Drawing for the job (mm, zero at the part's lowest x, y, z). A direction names the side the tool comes from. Give positions to 0.01 mm unless a question says otherwise; leave off trailing zeros. Loops run counter-clockwise (first coordinate to the right, second up) from the corner with the lowest first, then second, coordinate; pieces in that order, holes last. Notation, with made-up numbers: (20, 79.25) - (76, 79.25) arc R23 cw to (76, 117.25) - close; hole circle Ø2 at (34, 83.5). An arc over 180 degrees is marked (long way). Return JSON: item names as keys, results as strings. Group by question number.
1) Drop flat-ended pins along their axis: pin 1 (4 mm diameter, centred on x = 6, z = 9.5, fed in from -Y); pin 2 (3 mm diameter, centred on x = 3, y = 3.5, fed in from -Z); pin 3 (2 mm diameter, centred on x = 1, z = 9, fed in from -Y); pin 4 (2 mm diameter, centred on x = 2.5, z = 4.5, fed in from +Y). Give the stop position or say it passes through.
2) Drill centre lines: probe 1 along X at (y, z) = (4.5, 1.5); probe 2 along Z at (x, y) = (5.25, 5.75). Where is each one in solid material? Low to high. Write a range as from..to.
3) 3-axis set-ups, long thin cutter, end or side, ignore diameter. For the marked faces 1 and 2: which of +Z, -Z, +X, -X, +Y, -Y reach the whole face in a straight line?
4) Slice it at B-B (z = 9.5). List the corners of the cut face in (x, y), and give its area (3 significant figures).
5) Slice it at A-A (x = 3.5). List the corners of the cut face in (y, z), and give its area (3 significant figures).
6) Slice it at C-C (y = 2.75). List the corners of the cut face in (x, z), and give its area (3 significant figures).
7) Slice it at D-D (x = 6). List the corners of the cut face in (y, z).
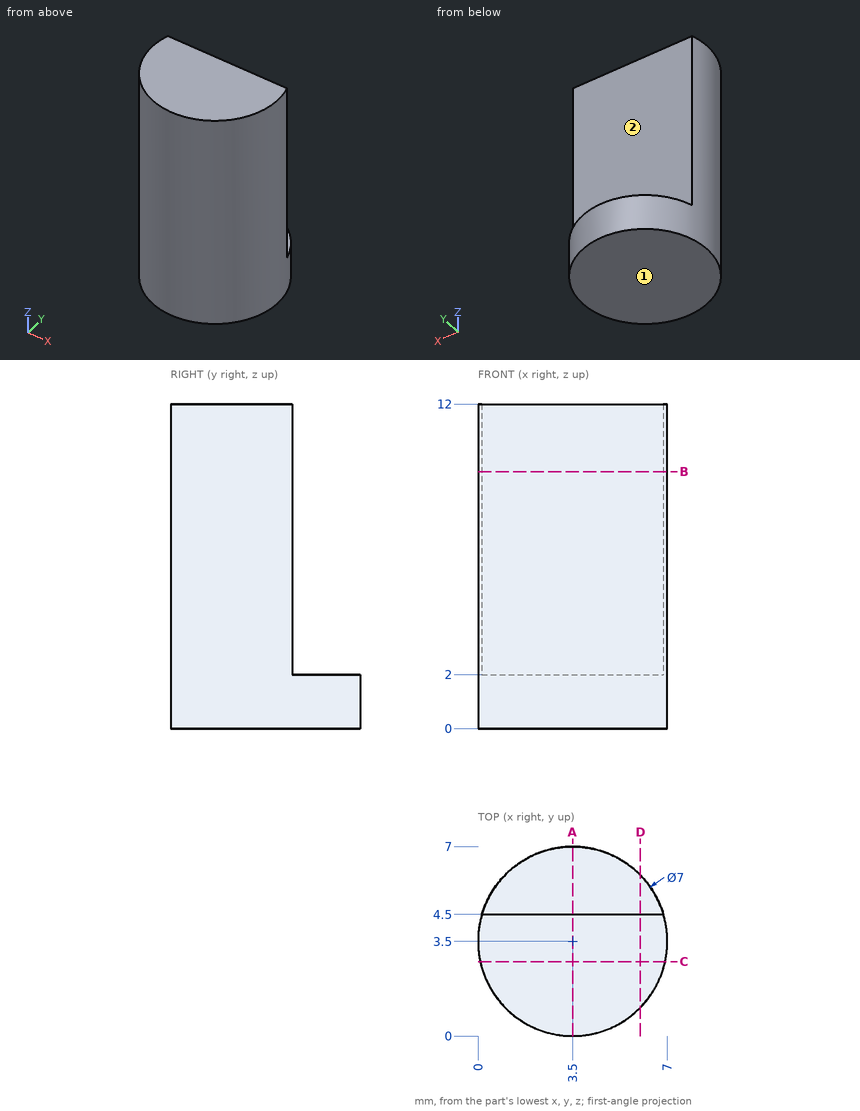
Results:
{
 "1": {"pin 1": "y = 0.04", "pin 2": "z = 0", "pin 3": "y = 0.34", "pin 4": "y = 4.5"},
 "2": {"probe 1": "0.15..6.85", "probe 2": "0..2"},
 "3": {"face 1": "-Z, +X, -X, +Y, -Y", "face 2": "+Z, +X, -X, +Y"},
 "4": {"outline": "(0.15, 4.5) arc R3.5 ccw (long way) to (6.85, 4.5) - close", "area": "26.1 mm2"},
 "5": {"outline": "(0, 0) - (7, 0) - (7, 2) - (4.5, 2) - (4.5, 12) - (0, 12) - close", "area": "59.0 mm2"},
 "6": {"outline": "(0.08, 0) - (6.92, 0) - (6.92, 12) - (0.08, 12) - close", "area": "82.0 mm2"},
 "7": {"outline": "(1.05, 0) - (5.95, 0) - (5.95, 2) - (4.5, 2) - (4.5, 12) - (1.05, 12) - close"}
}
